```python
from build123d import *

# Parameters (mm, degrees)
BOSS_EXTRUDE1_DEPTH = 200
SKETCH2_W           = 29.8
SKETCH2_H           = 9.8
BOSS_EXTRUDE2_DEPTH = 30
FILLET1_R           = 10
FILLET2_R           = 10
CUT_EXTRUDE1_DEPTH  = 56


with BuildPart() as part:
    # Sketch1 → Boss-Extrude1 (new body)
    with BuildSketch(Plane.XY):
        Polygon((0, 0), (14.9, 0), (14.9, 9.8), (-14.9, 9.8), (-14.9, 0), align=None)
    extrude(amount=-BOSS_EXTRUDE1_DEPTH)

    # Sketch2 → Boss-Extrude2 (add)
    with BuildSketch(Plane.XY.offset(-5)):
        with BuildLine():
            ThreePointArc((-25.1, -10), (-24.221320344, -12.121320344), (-22.1, -13))
            ThreePointArc((-22.1, -13), (-21.670577963, -12.969107057), (-21.25, -12.877064476))
            ThreePointArc((-21.25, -12.877064476), (0, -9.80367638), (21.25, -12.877064476))
            ThreePointArc((21.25, -12.877064476), (21.670577963, -12.969107057), (22.1, -13))
            ThreePointArc((22.1, -13), (24.221320344, -12.121320344), (25.1, -10))
            Line((25.1, -10), (25.1, 6.8))
            ThreePointArc((25.1, 6.8), (22.171067812, 13.871067812), (15.1, 16.8))
            Line((15.1, 16.8), (-14.9, 16.8))
            Line((-14.9, 16.8), (-15.1, 16.8))
            ThreePointArc((-15.1, 16.8), (-22.171067812, 13.871067812), (-25.1, 6.8))
            Line((-25.1, 6.8), (-25.1, -10))
        make_face()
        with Locations((0, 4.9)):
            Rectangle(SKETCH2_W, SKETCH2_H, mode=Mode.SUBTRACT)
    extrude(amount=-BOSS_EXTRUDE2_DEPTH)

    # Fillet1
    # the kernel refuses this fillet: 10 mm, written as the material it takes off along each edge
    with BuildSketch(Plane(origin=(14.9, -21.650635095, 0), x_dir=(0, 0, -1), z_dir=(0, 1, 0))) as fillet1_piece_1:
        with BuildLine():
            CenterArc((10, 8.660254038), FILLET1_R, 180, 60)
            Line((0, 8.660254038), (-0.2, 8.660254038))
            Line((-0.2, 8.660254038), (-0.2, 0))
            Line((-0.2, 0), (0, -0.2))
            ThreePointArc((0, -0.2), (2.5, -0.2), (4.9, -0.173205081))
            Line((4.9, -0.173205081), (5, 0))
        make_face()
    extrude(amount=53.101270189, mode=Mode.SUBTRACT)

    # Fillet2
    # the kernel refuses this fillet: 10 mm, written as the material it takes off along each edge
    with BuildSketch(Plane(origin=(-14.9, 31.450635095, 0), x_dir=(1, 0, 0), z_dir=(0, -1, 0))) as fillet2_piece_1:
        with BuildLine():
            CenterArc((8.660254038, -10), FILLET2_R, 90, 60)
            Line((0, -5), (-0.173205081, -4.9))
            ThreePointArc((-0.173205081, -4.9), (-0.2, -2.5), (-0.2, 0))
            Line((-0.2, 0), (0, 0.2))
            Line((0, 0.2), (8.660254038, 0.2))
            Line((8.660254038, 0.2), (8.660254038, 0))
        make_face()
    extrude(amount=53.101270189, mode=Mode.SUBTRACT)

    # Sketch3 → Cut-Extrude1 (cut)
    with BuildSketch(Plane(origin=(25.1, 0, 0), x_dir=(0, 0, -1), z_dir=(1, 0, 0))):
        Polygon((30, -4), (30, -8), (20, -8), (10, -8), (10, -4), align=None)
    extrude(amount=-CUT_EXTRUDE1_DEPTH, mode=Mode.SUBTRACT)


solid = part.part
```
Check sheet for the modelled part. Datum: model origin and axes. Units: mm. A direction names the side the tool comes from. Round coordinates to 2 decimals unless told otherwise and drop trailing zeros. Order: outer loops, then holes, each group sorted by start corner. A loop starts at its lowest first (then second) coordinate and runs counter-clockwise, first axis right, second up. Notation, with made-up numbers: (34.25, 54.25) -> (88.25, 54.25) arc R21 cw to (88.25, 93.25) -> close; hole circle Ø2 at (-24.5, 6.5). An arc over 180 degrees is marked (long way). One line per item, written item: value. Start each with the question number.
Q1. Mould release check, pull along X, two halves, no side actions. Record for faces 1 (the face through (11.176, 4.831, -1.303)), 2 (the face through (0, 9.8, -2)), 3 (the face through (-11.176, 4.969, -1.303)), 4 (the face through (-0.302, -9.804, -19.79)): pulls with the +X half, pulls with the -X half, needs draft (parallel to the pull), parting line crosses it, or undercut.
Q2. Set-up check for faces 5 (the face through (0, 0, -2)), 6 (the face through (0, -6, -10)), 7 (the face through (14.9, 5, -116)), 8 (the face through (0, 9.8, -116)): record each of +Z, -Z, +X, -X, +Y, -Y from which the full face is reachable in a straight line by a thin tool's end or side.
Q3. Cross-section at D-D (x = 8). Record the boundary of the cut face in (y, z), and give its area (3 significant figures).
Q4. Gauge pin test, flat ends, axial feed: pin 1 Ø16 at (x, z) = (5.5, -21) entering from -Y; pin 2 Ø8 at (y, z) = (12, -107.5) entering from +X; pin 3 Ø10 at (x, y) = (-16.5, 12.5) entering from +Z. Record the tip position at first contact, or that the pin passes through.
Q5. Cross-section at A-A (x = 0). Record the boundary of the cut face in (y, z).
Q6. Cross-section at C-C (z = -45). Record the boundary of the cut face in (x, y), and give its area (3 significant figures).
Q7. Cross-section at B-B (y = 4). Record the boundary of the cut face in (x, z), and give its area (3 significant figures).
Q8. Thickness scan on line 1 (Z direction, x = 7, y = -7.5); line 2 (X direction, y = 6.75, z = -123.5); line 3 (Z direction, x = 14.5, y = 10.5). Record the ranges inside material, lowest first.
Completed:
1. face 1: pulls with the +X half
1. face 2: needs draft
1. face 3: pulls with the -X half
1. face 4: undercut
2. face 5: +Z, +X, -X, -Y
2. face 6: +X, -X
2. face 7: -Z, +X, +Y, -Y
2. face 8: -Z, +X, -X, +Y
3. outline: (-10.23, -35) -> (0, -35) -> (0, -200) -> (9.8, -200) -> (9.8, -35) -> (16.8, -35) -> (16.8, -5) -> (9.8, -5) -> (9.8, -0.16) -> (0, -0.16) -> (0, -5) -> (-10.23, -5) -> close; hole (-8, -30) -> (-4, -30) -> (-4, -10) -> (-8, -10) -> close
3. area: 2,400 mm²
4. pin 1: stops at y = -11.03
4. pin 2: stops at x = 14.9
4. pin 3: stops at z = -2.04
5. outline: (-9.8, -35) -> (0, -35) -> (0, -200) -> (9.8, -200) -> (9.8, -35) -> (16.8, -35) -> (16.8, -5) -> (9.8, -5) -> (9.8, 0) -> (0, 0) -> (0, -5) -> (-9.8, -5) -> close; hole (-8, -30) -> (-4, -30) -> (-4, -10) -> (-8, -10) -> close
6. outline: (-14.9, 0) -> (14.9, 0) -> (14.9, 9.8) -> (-14.9, 9.8) -> close
6. area: 292 mm²
7. outline: (-25.1, -35) -> (-14.9, -35) -> (-14.9, -200) -> (14.9, -200) -> (14.9, -35) -> (25.1, -35) -> (25.1, -5) -> (14.9, -5) arc R10 ccw to (6.24, 0) -> (-6.24, 0) arc R10 ccw to (-14.9, -5) -> (-25.1, -5) -> close
7. area: 6,550 mm²
8. line 1: z = -35 to -30, -10 to -5
8. line 2: x = -14.9 to 14.9
8. line 3: z = -35 to -5
